Geometry check sheet. Reference: drawing and pictorial views, mm from the part's lowest x, y, z. A direction names the side the tool comes from. Give positions to 0.01 mm unless a question says otherwise; leave off trailing zeros. Order: outer loops, then holes, each group sorted by start corner. A loop starts at its lowest first (then second) coordinate and runs counter-clockwise, first axis right, second up.
Item 1: Material ranges on line 1 along X through (y, z) = (4.5, 6.5); line 2 along Y through (x, z) = (10.75, 10.75); line 3 along Y through (x, z) = (6, 0.95), recorded low to high.
Item 2: Sectioned sample at A-A on z = 12.5. Record the boundary of the cut face in (x, y).
Item 3: Release check for a two-part mould opening along Y. For the marked faces 1, 2 and 3 record: released by +Y, released by -Y, zero draft, split by the parting line, or undercut.
Item 4: Sectioned sample at B-B on x = 6. Record the boundary of the cut face in (y, z), and give its area (4 significant figures).
Item 5: Sectioned sample at C-C on z = 2.5. Record the boundary of the cut face in (x, y).
Item 6: Access from +Z, -Z, +X, -X, +Y, -Y to the whole of each face (thin tool, end or side, straight path). Record for the marked faces 4, 5 and 6.
Item 7: Sectioned sample at D-D on y = 5.85. Record the boundary of the cut face in (x, z), and give its area (3 significant figures).
Item 8: Gauge pin test, flat ends, axial feed: P1, Ø0.8, axis at x = 11.5, y = 6.5, coming from the +Z side; P2, Ø5, axis at x = 6.5, z = 9, coming from the +Y side; P3, Ø1, axis at x = 3.5, y = 6.5, coming from the +Z side. Record the tip position at first contact, or that the pin passes through.
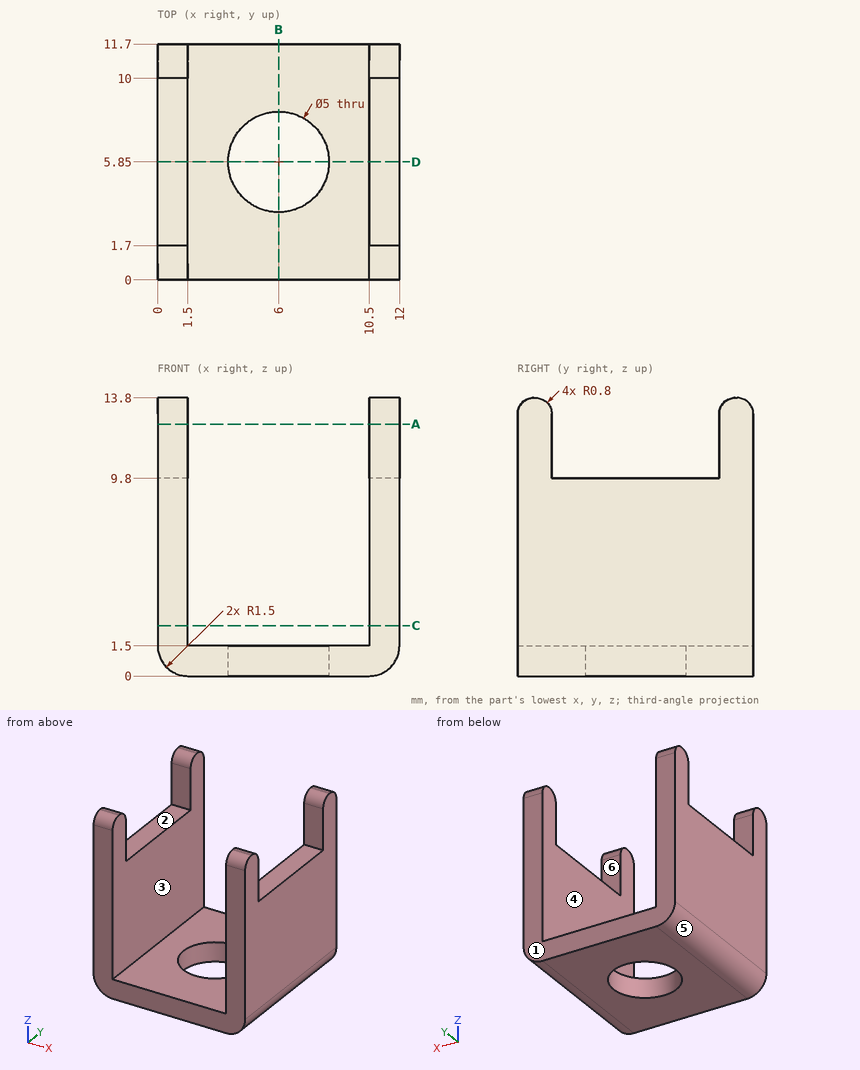
Report:
1. line 1: x = 0 to 1.5, 10.5 to 12
1. line 2: y = 0 to 1.7, 10 to 11.7
1. line 3: y = 0 to 3.35, 8.35 to 11.7
2. outline: (0, 0) - (1.5, 0) - (1.5, 1.7) - (0, 1.7) - close; (0, 10) - (1.5, 10) - (1.5, 11.7) - (0, 11.7) - close; (10.5, 0) - (12, 0) - (12, 1.7) - (10.5, 1.7) - close; (10.5, 10) - (12, 10) - (12, 11.7) - (10.5, 11.7) - close
3. face 1: released by +Y
3. face 2: undercut
3. face 3: zero draft
4. outline: (0, 0) - (3.35, 0) - (3.35, 1.5) - (0, 1.5) - close; (8.35, 0) - (11.7, 0) - (11.7, 1.5) - (8.35, 1.5) - close
4. area: 10.05 mm2
5. outline: (0, 0) - (1.5, 0) - (1.5, 11.7) - (0, 11.7) - close; (10.5, 0) - (12, 0) - (12, 11.7) - (10.5, 11.7) - close
6. face 4: +Z, +Y, -Y
6. face 5: -Z, -X, +Y, -Y
6. face 6: +Z, +X, -X
7. outline: (0, 1.5) arc R1.5 ccw to (1.5, 0) - (3.5, 0) - (3.5, 1.5) - (1.5, 1.5) - (1.5, 9.8) - (0, 9.8) - close; (8.5, 0) - (10.5, 0) arc R1.5 ccw to (12, 1.5) - (12, 9.8) - (10.5, 9.8) - (10.5, 1.5) - (8.5, 1.5) - close
7. area: 34.4 mm2
8. P1: stops at z = 9.8
8. P2: passes through
8. P3: stops at z = 1.5
